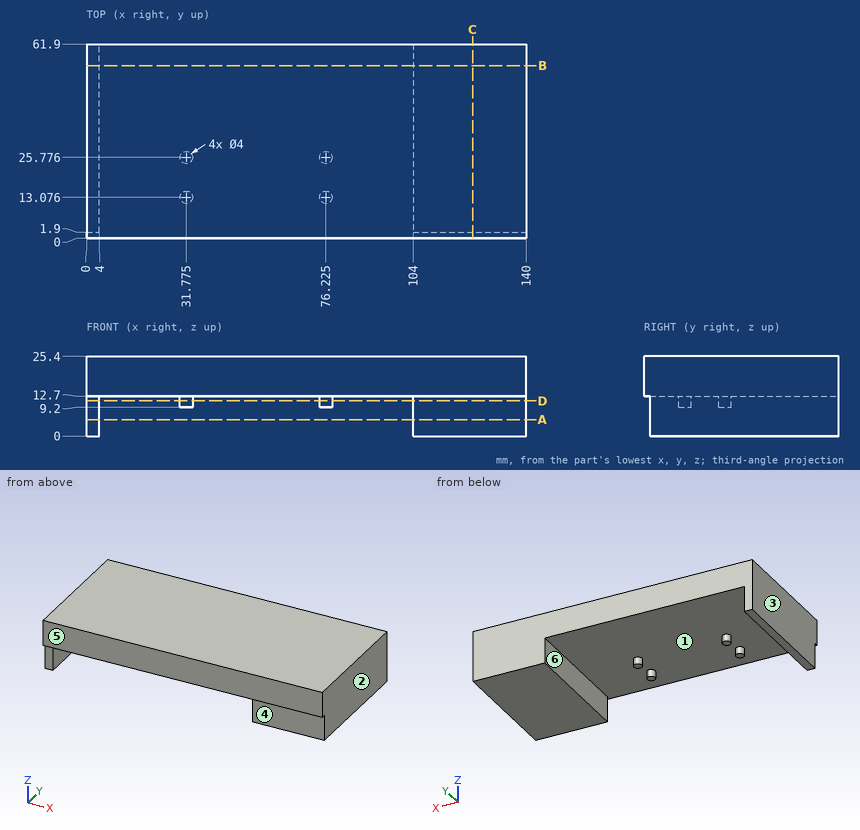
Source: three-view drawing plus pictorial views. Frame: mm from the lowest corner of the part. A direction names the side the tool comes from. Round coordinates to 2 decimals unless told otherwise and drop trailing zeros. Loops run counter-clockwise (first coordinate to the right, second up) from the corner with the lowest first, then second, coordinate; pieces in that order, holes last.
1. Section query C-C on x = 123. Output: boundary loops of the cut face in (y, z), and give its area (3 significant figures).
2. Section query B-B on y = 55. Output: boundary loops of the cut face in (x, z), and give its area (3 significant figures).
3. Access query for the marked faces 5 and 6. Directions: +Z, -Z, +X, -X, +Y, -Y. A direction counts if a zero-diameter tool reaches every point of the face in a straight line with its end or side. Return the directions, or none.
4. Contact query for flat-ended pins moving along their axis: pin 1 (1.2 mm diameter, centred on x = 77, y = 12.5, fed in from -Z); pin 2 (6.5 mm diameter, centred on x = 128, z = 3.5, fed in from -Y); pin 3 (10 mm diameter, centred on x = 95, y = 34.5, fed in from -Z). Output: stop coordinate, or through.
5. Ray query, L1, parallel to X at y = 27.5, z = 4.75; L2, parallel to X at y = 24, z = 12; L3, parallel to Z at x = 83.5, y = 4. Return the intervals inside material, ascending.
6. Section query D-D on z = 11.25. Output: boundary loops of the cut face in (x, y) (3 decimals).
7. Mould query, pull axis X, two halves, no side actions, for the marked faces 1, 2, 3 and 4. Classes: released by +X, released by -X, zero draft, split by the parting line, or undercut.
8. Section query A-A on z = 5.25. Output: boundary loops of the cut face in (x, y), and give its area (3 significant figures).
Answers below:
1. outline: (0, 12.7) - (1.9, 12.7) - (1.9, 0) - (61.9, 0) - (61.9, 25.4) - (0, 25.4) - close
1. area: 1,550 mm2
2. outline: (0, 0) - (4, 0) - (4, 12.7) - (104, 12.7) - (104, 0) - (140, 0) - (140, 25.4) - (0, 25.4) - close
2. area: 2,290 mm2
3. face 5: +Z, -Z, +X, -X, -Y
3. face 6: -Z, +Y, -Y
4. pin 1: stops at z = 9.2
4. pin 2: stops at y = 1.9
4. pin 3: stops at z = 12.7
5. L1: x = 0 to 4, 104 to 140
5. L2: x = 0 to 4, 30.86 to 32.69, 75.31 to 77.14, 104 to 140
5. L3: z = 12.7 to 25.4
6. outline: (0, 1.9) - (4, 1.9) - (4, 61.9) - (0, 61.9) - close; circle Ø4 at (31.775, 13.076); circle Ø4 at (31.775, 25.776); circle Ø4 at (76.225, 13.076); circle Ø4 at (76.225, 25.776); (104, 1.9) - (140, 1.9) - (140, 61.9) - (104, 61.9) - close
7. face 1: undercut
7. face 2: released by +X
7. face 3: released by -X
7. face 4: zero draft
8. outline: (0, 1.9) - (4, 1.9) - (4, 61.9) - (0, 61.9) - close; (104, 1.9) - (140, 1.9) - (140, 61.9) - (104, 61.9) - close
8. area: 2,400 mm2
